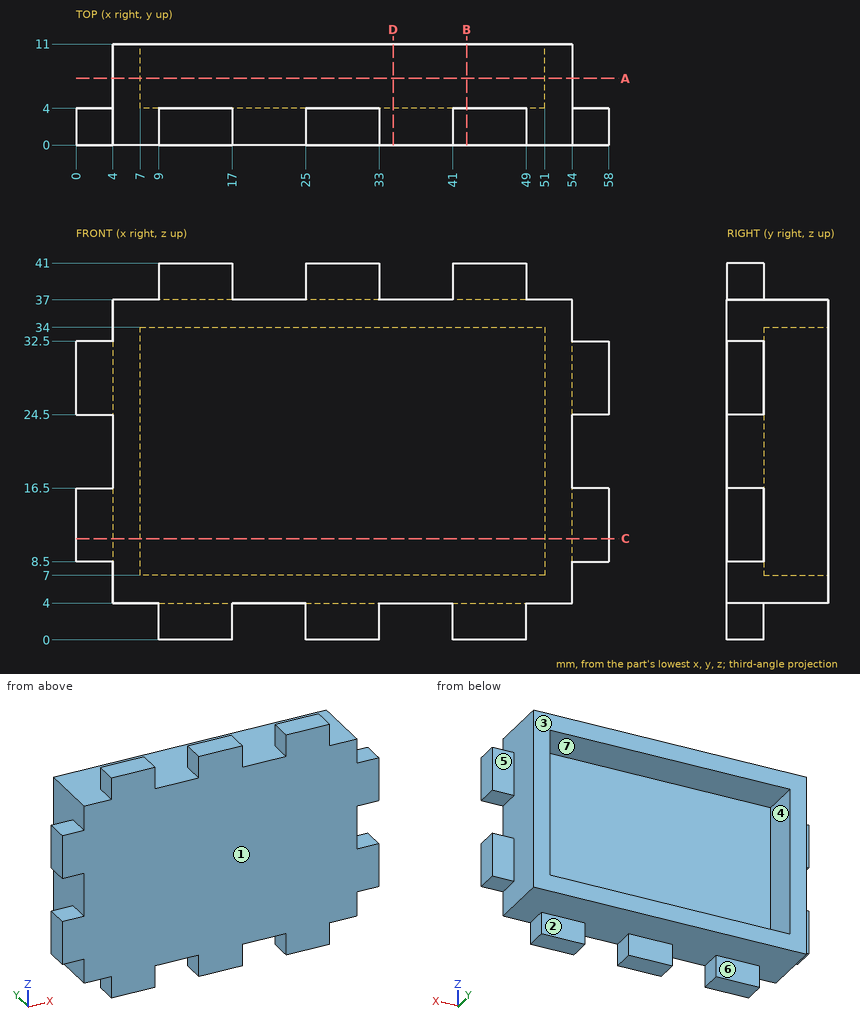
Here's the drawing with two shaded views (mm, measured from the low corner). I have some questions. A direction names the side the tool comes from. Round coordinates to 2 decimals unless told otherwise and drop trailing zeros. Loops run counter-clockwise (first coordinate to the right, second up) from the corner with the lowest first, then second, coordinate; pieces in that order, holes last.
1. Suppose I cut it at A-A, the plane y = 7.25. Please give me the cut outline in (x, z).
Answers:
outline: (4, 4) - (54, 4) - (54, 37) - (4, 37) - close; hole (7, 7) - (51, 7) - (51, 34) - (7, 34) - close
2. Will these pins go through, and if not, where does the flat tip stop? pin 1 (4.5 mm diameter, centred on x = 57, y = 3, fed in from +Z); pin 2 (3 mm diameter, centred on x = 56.5, z = 28.5, fed in from +Y); pin 3 (4.5 mm diameter, centred on x = 3, y = 2, fed in from +Z); pin 4 (3 mm diameter, centred on y = 3, z = 9, fed in from -X).
Answers:
pin 1: stops at z = 32.5
pin 2: stops at y = 4
pin 3: stops at z = 37
pin 4: stops at x = 0
3. Suppose I cut it at B-B, the plane x = 42.5. Please give me the cut outline in (y, z).
Answers:
outline: (0, 0) - (4, 0) - (4, 4) - (11, 4) - (11, 7) - (4, 7) - (4, 34) - (11, 34) - (11, 37) - (4, 37) - (4, 41) - (0, 41) - close
4. Suppose I cut it at C-C, the plane z = 11. Please give me the cut outline in (x, y), and give its area (3 significant figures).
Answers:
outline: (0, 0) - (58, 0) - (58, 4) - (54, 4) - (54, 11) - (51, 11) - (51, 4) - (7, 4) - (7, 11) - (4, 11) - (4, 4) - (0, 4) - close
area: 274 mm2
5. If I drill on probe 1 along Z at (x, y) = (35.5, 8.5); probe 2 along X at (y, z) = (10.75, 32.5); probe 3 along X at (y, z) = (4, 35), over which ranges is the centre line in solid material (lowest first)?
Answers:
probe 1: z = 4 to 7, 34 to 37
probe 2: x = 4 to 7, 51 to 54
probe 3: x = 4 to 54
6. Thinking about a two-plate mould opening in X: for the marked faces 6 and 7, which applies, released by +X, released by -X, zero draft, split by the parting line, or undercut?
Answers:
face 6: zero draft
face 7: undercut
7. For the marked faces 1, 2, 3, 4 and 5, which set-ups out of +Z, -Z, +X, -X, +Y, -Y let a thin tool reach every point of the face, with its end or its side?
Answers:
face 1: +Z, -Z, +X, -X, -Y
face 2: -Z, +X, -X, +Y
face 3: +Z, -Z, +X, -X, +Y
face 4: +Y
face 5: +Z, -Z, +X, +Y
8. Suppose I cut it at D-D, the plane x = 34.5. Please give me the cut outline in (y, z), and give its area (3 significant figures).
Answers:
outline: (0, 4) - (11, 4) - (11, 7) - (4, 7) - (4, 34) - (11, 34) - (11, 37) - (0, 37) - close
area: 174 mm2
